The model under review builds one solid part; all positions refer to its coordinate system, in mm. Face numbers are marked on the shaded views. Coordinates: 2 decimals unless noted, no trailing zeros. Loops run counter-clockwise (first coordinate to the right, second up) from the corner with the lowest first, then second, coordinate; pieces in that order, holes last. Notation, with made-up numbers: M 60.25,81 L 104.25,81 A20 ccw 104.25,117 Z; hole C 34.25,69 d9. An arc over 180 degrees is marked long. One line per item, written item: value.
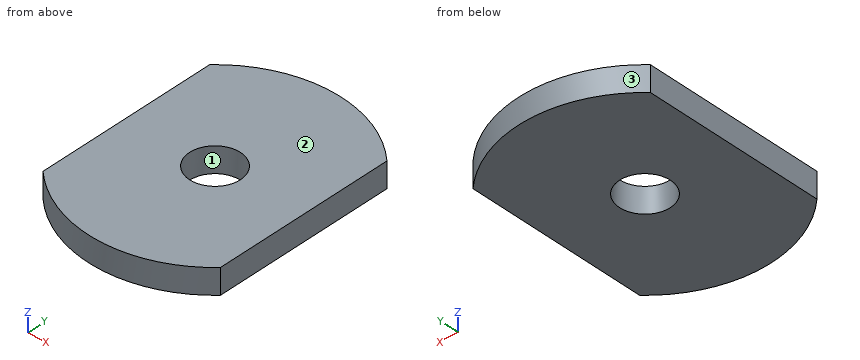
```python
from build123d import *

# Parameters (mm, degrees)
F0_R     = 63.5
F0_R_2   = 12.7
F1_DEPTH = 12.7
F3_W     = 54.029742
F3_H     = 140.439012
F3_W_2   = 66.675002
F3_H_2   = 141.013797
F4_DEPTH = 25.4


with BuildPart() as f1:
    # F0 (on Top) → F1 (new body)
    with BuildSketch(Plane.XY):
        Circle(F0_R)
        Circle(F0_R_2, mode=Mode.SUBTRACT)
    extrude(amount=F1_DEPTH)

    # F3 (on face) → F4 (cut)
    with BuildSketch(Plane.XY.offset(12.7)):
        with Locations((-71.464871, -3.700142)):
            Rectangle(F3_W, F3_H)
        with Locations((77.787501, -3.412749)):
            Rectangle(F3_W_2, F3_H_2)
    extrude(amount=-F4_DEPTH, mode=Mode.SUBTRACT)


solid = f1.part
```
(1) Draft analysis for pull direction Y (two halves, no side actions). For the marked faces 1, 2 and 3, state which applies: pulls with the +Y half, pulls with the -Y half, needs draft (parallel to the pull), parting line crosses it, or undercut.
Checks:
face 1: undercut
face 2: needs draft
face 3: pulls with the +Y half
(2) Add section B-B on x = 0. State the section outline as (y, z) points.
Checks:
outline: M -63.5,0 L -12.7,0 L -12.7,12.7 L -63.5,12.7 Z; M 12.7,0 L 63.5,0 L 63.5,12.7 L 12.7,12.7 Z
(3) Add section D-D on x = -34.5. State the section outline as (y, z) points, then the cut area to 3 significant figures.
Checks:
outline: M -53.31,0 L 53.31,0 L 53.31,12.7 L -53.31,12.7 Z
area: 1,350 mm^2
(4) To check wall thickness, follow L1, parallel to Y at x = 0, z = 7; L2, parallel to Y at x = -3.5, z = 12.25; L3, parallel to X at y = 6, z = 1.25. State the ranges of each line that lie inside material, in increasing order. Write a range as [from, to].
Checks:
L1: [-63.5, -12.7], [12.7, 63.5]
L2: [-63.4, -12.21], [12.21, 63.4]
L3: [-44.45, -11.19], [11.19, 44.45]
(5) Add section C-C on z = 2. State the section outline as (x, y) points, then the cut area to 3 significant figures.
Checks:
outline: M -44.45,-45.35 A63.5 ccw 44.45,-45.35 L 44.45,45.35 A63.5 ccw -44.45,45.35 Z; hole C 0,0 d25.4
area: 9,780 mm^2
(6) Add section A-A on y = 0. State the section outline as (x, z) points, then the cut area to 3 significant figures.
Checks:
outline: M -44.45,0 L -12.7,0 L -12.7,12.7 L -44.45,12.7 Z; M 12.7,0 L 44.45,0 L 44.45,12.7 L 12.7,12.7 Z
area: 806 mm^2
(7) Insertion check: pin 1 Ø1 at (x, z) = (-14.5, 2) entering from +Y; pin 2 Ø4 at (x, z) = (9.5, 3.5) entering from +Y; pin 3 Ø1 at (x, y) = (-28.5, 47.5) entering from -Z; pin 4 Ø5 at (x, z) = (18, 10) entering from +Y. Each pin has a flat end and moves straight along its axis. Give the tip position at first contact, or say it passes through.
Checks:
pin 1: y = 61.94
pin 2: y = 63.06
pin 3: z = 0
pin 4: y = 61.58
